CAD build for the part. Positions are in the model's coordinates, mm. Face numbers are marked on the shaded views. A direction names the side the tool comes from. Round coordinates to 2 decimals unless told otherwise and drop trailing zeros. Loops run counter-clockwise (first coordinate to the right, second up) from the corner with the lowest first, then second, coordinate; pieces in that order, holes last.
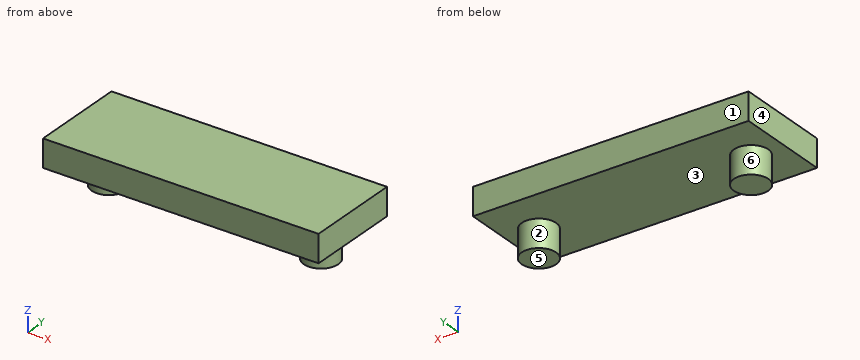
Autodesk Inventor part; units mm, degrees
ref_plane "YZ Plane" through (0, 0, 0) normal (1, 0, 0) x (0, 1, 0)
ref_plane "XZ Plane" through (0, 0, 0) normal (0, 1, 0) x (-1, 0, 0)
ref_plane "XY Plane" through (0, 0, 0) normal (0, 0, 1) x (1, 0, 0)
sketch "Sketch5" plane through (0, 0, 0) normal (0, 0, 1) x (1, 0, 0)
  line L0 (7, -1.5) -> (0.5048, -1.5)
  circle A0 centre (14.7, 0) radius 1.25
  circle A1 centre (-0.7, 0) radius 1.25
  line L1 (-3, -3.5) -> (17, -3.5)
  line L2 (17, -3.5) -> (17, 3.5)
  line L3 (17, 3.5) -> (-3, 3.5)
  line L4 (-3, 3.5) -> (-3, -3.5)
  point P0 (0, 0)
extrude "Extrusion7" add sketch "Sketch5" along normal blind 2 contours A0 | A1 | L4 L3 L2 L1
extrude "Extrusion8" add sketch "Sketch5" against normal blind 2 contours A0 | A1
properties part number "test_izbrisi"
Item 1: Two-plate mould, pull along X, no slides. Class the marked faces 1, 2, 3 and 4: released by +X, released by -X, zero draft, split by the parting line, or undercut.
Answers follow:
face 1: zero draft
face 2: undercut
face 3: undercut
face 4: released by -X
Item 2: Flat gauge pin, fed straight in: P1, Ø2, axis at y = -1, z = -1.5, coming from the -X side. Where does the tip first touch, or does it go through?
Answers follow:
P1: stops at x = -1.95
Item 3: Cut at A-A, the plane y = 0. Give the cut face in (x, z), plus the area to 3 significant figures.
Answers follow:
outline: (-3, 0) - (-1.95, 0) - (-1.95, -2) - (0.55, -2) - (0.55, 0) - (13.45, 0) - (13.45, -2) - (15.95, -2) - (15.95, 0) - (17, 0) - (17, 2) - (-3, 2) - close
area: 50.0 mm2
Item 4: Cut at C-C, the plane z = -0.9. Give the cut face in (x, y), plus the area to 3 significant figures.
Answers follow:
outline: circle Ø2.5 at (-0.7, 0); circle Ø2.5 at (14.7, 0)
area: 9.82 mm2
Item 5: 3-axis set-ups, long thin cutter, end or side, ignore diameter. For the marked faces 5 and 6: which of +Z, -Z, +X, -X, +Y, -Y reach the whole face in a straight line?
Answers follow:
face 5: -Z, +X, -X, +Y, -Y
face 6: -Z
Item 6: Probe line 1 (Z direction, x = 12.5, y = 0); line 2 (X direction, y = -0.75, z = -1); line 3 (X direction, y = 0.5, z = -1.55). List the from-to ranges inside material, lowest first.
Answers follow:
line 1: z = 0 to 2
line 2: x = -1.7 to 0.3, 13.7 to 15.7
line 3: x = -1.85 to 0.45, 13.55 to 15.85
Item 7: Cut at B-B, the plane x = 14.7. Give the cut face in (y, z).
Answers follow:
outline: (-3.5, 0) - (-1.25, 0) - (-1.25, -2) - (1.25, -2) - (1.25, 0) - (3.5, 0) - (3.5, 2) - (-3.5, 2) - close
Item 8: Cut at D-D, the plane y = 2.5. Give the cut face in (x, z).
Answers follow:
outline: (-3, 0) - (17, 0) - (17, 2) - (-3, 2) - close
